```python
from build123d import *

# Parameters (mm, degrees)
ESQUISSE1_R        = 1.9
ESQUISSE1_W        = 3
ESQUISSE1_H        = 12
BOSS_EXTRU_1_DEPTH = 5


with BuildPart() as part:
    # Esquisse1 → Boss.-Extru.1 (new body)
    with BuildSketch(Plane.XY):
        with BuildLine():
            Line((-6.95859236, 59.924430221), (3.04140764, 59.924430221))
            ThreePointArc((3.04140764, 59.924430221), (6.576941546, 58.459964127), (8.04140764, 54.924430221))
            Line((8.04140764, 54.924430221), (8.04140764, 43.659711595))
            ThreePointArc((8.04140764, 43.659711595), (7.584684835, 41.363611001), (6.284048327, 39.417070908))
            Line((6.284048327, 39.417070908), (5.227699141, 38.360721722))
            ThreePointArc((5.227699141, 38.360721722), (1.75933512, 33.169948141), (0.54140764, 27.047013223))
            Line((0.54140764, 27.047013223), (0.54140764, -52.575569779))
            ThreePointArc((0.54140764, -52.575569779), (-5.70859236, -58.825569779), (-11.95859236, -52.575569779))
            Line((-11.95859236, -52.575569779), (-11.95859236, 54.924430221))
            ThreePointArc((-11.95859236, 54.924430221), (-10.494126266, 58.459964127), (-6.95859236, 59.924430221))
        make_face()
        with Locations((-5.70859236, -52.575569779)):
            Circle(ESQUISSE1_R, mode=Mode.SUBTRACT)
        with Locations((3.04140764, 52.424430221)):
            Circle(ESQUISSE1_R, mode=Mode.SUBTRACT)
        with Locations((-6.95859236, 52.424430221)):
            Circle(ESQUISSE1_R, mode=Mode.SUBTRACT)
        with Locations((-5.70859236, 17.424430221)):
            Rectangle(ESQUISSE1_W, ESQUISSE1_H, mode=Mode.SUBTRACT)
        with Locations((-5.70859236, -20.575569779)):
            Rectangle(ESQUISSE1_W, ESQUISSE1_H, mode=Mode.SUBTRACT)
    extrude(amount=BOSS_EXTRU_1_DEPTH)


solid = part.part
```
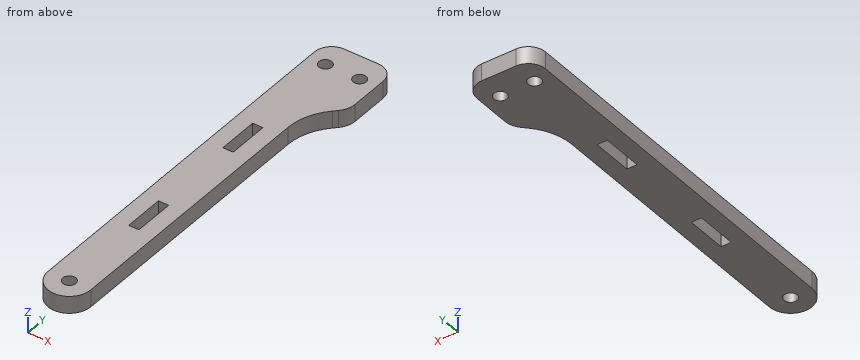
For this review, take the finished solid that the model builds, in its own axes (mm). Coordinates: 2 decimals unless noted, no trailing zeros. Loops run counter-clockwise (first coordinate to the right, second up) from the corner with the lowest first, then second, coordinate; pieces in that order, holes last.
1. Add section B-B, the plane z = 3.1. Give the boundary of the cut face in (x, y), then the cut area to 3 significant figures.
2. Add section A-A, the plane y = 17. Give the boundary of the cut face in (x, z).
3. Insertion check: P1, Ø1.5, axis at y = -7, z = 2.5, coming from the +X side; P2, Ø1.5, axis at y = 31, z = 2.5, coming from the +X side; P3, Ø3, axis at x = -9.5, z = 4.5, coming from the -Y side. Each pin has a flat end and moves straight along its axis. Give the tip position at first contact, or say it passes through.
4. For line 1 (X direction, y = 52.5, z = 2.5); line 2 (X direction, y = -23, z = 2.65); line 3 (Y direction, x = -7, z = 2.3), list the stretches that pass through material, from the lowest coordinate up.
5. Add section D-D, the plane y = -7. Give the boundary of the cut face in (x, z).
6. Add section C-C, the plane x = -0.5. Give the boundary of the cut face in (y, z), then the cut area to 3 significant figures.
Result:
1. outline: (-11.96, -52.58) arc R6.25 ccw to (0.54, -52.58) - (0.54, 27.05) arc R16 cw to (5.23, 38.36) - (6.28, 39.42) arc R6 ccw to (8.04, 43.66) - (8.04, 54.92) arc R5 ccw to (3.04, 59.92) - (-6.96, 59.92) arc R5 ccw to (-11.96, 54.92) - close; hole circle Ø3.8 at (-6.96, 52.42); hole circle Ø3.8 at (-5.71, -52.58); hole (-7.21, -26.58) - (-4.21, -26.58) - (-4.21, -14.58) - (-7.21, -14.58) - close; hole (-7.21, 11.42) - (-4.21, 11.42) - (-4.21, 23.42) - (-7.21, 23.42) - close; hole circle Ø3.8 at (3.04, 52.42)
1. area: 1,520 mm2
2. outline: (-11.96, 0) - (-7.21, 0) - (-7.21, 5) - (-11.96, 5) - close; (-4.21, 0) - (0.54, 0) - (0.54, 5) - (-4.21, 5) - close
3. P1: stops at x = 0.54
3. P2: stops at x = 1.25
3. P3: stops at y = -58.39
4. line 1: x = -11.96 to -8.86, -5.06 to 1.14, 4.94 to 8.04
4. line 2: x = -11.96 to -7.21, -4.21 to 0.54
4. line 3: y = -58.69 to -53.97, -51.18 to -26.58, -14.58 to 11.42, 23.42 to 50.52, 54.32 to 59.92
5. outline: (-11.96, 0) - (0.54, 0) - (0.54, 5) - (-11.96, 5) - close
6. outline: (-56.03, 0) - (59.92, 0) - (59.92, 5) - (-56.03, 5) - close
6. area: 580 mm2
